Could you check a few things on this model? Use its own coordinates, in mm. Coordinates: 2 decimals unless noted, no trailing zeros. Loops run counter-clockwise (first coordinate to the right, second up) from the corner with the lowest first, then second, coordinate; pieces in that order, holes last. Notation, with made-up numbers: M 56.25,89.5 L 69.25,89.5 A31 ccw 69.25,120.5 Z; hole C 88.25,33 d3. An arc over 180 degrees is marked long. Use one line per item in the form item = value. Start each with the question number.
Autodesk Fusion 360 part; units mm, degrees
box "BoxPrimitive1" add length 123 width 170 height 1 placed x (0, -1, 0) y (1, 0, 0) z (0, 0, 1) at (0, 0, 0) makes body 1
cylinder "CylinderPrimitive1" add diameter 5 height 10 placed x (0, 0, -1) y (0, 1, 0) z (1, 0, 0) at (0, 10, 10) separate body makes body 2
move_body "Move1" bodies 2 to x (1, 0, 0) y (0, 1, 0) z (0, 0, 1) at (0, -10, -10)
move_body "Move2" bodies 2 to x (1, 0, 0) y (0, 1, 0) z (0, 0, 1) at (0, -61.5, 0)
move_body "Move3" bodies 2 to x (1, 0, 0) y (0, 1, 0) z (0, 0, 1) at (-5, 0, 0)
combine "Combine1" operation add target body 1 tool bodies 2
cylinder "CylinderPrimitive2" cut diameter 3.5 height -1 placed x (1, 0, 0) y (0, 1, 0) z (0, 0, 1) at (24, -14, 1) bodies 1
Item 1: Thinking about a two-plate mould opening in Y: for faces 1 (the cylindrical face through (22.71, -12.82, 0.51)), 2 (the flat face through (86, -61, 1)), 3 (the cylindrical face through (0.07, -60.749, -2.385)), which applies, pulls with the +Y half, pulls with the -Y half, needs draft (parallel to the pull), parting line crosses it, or undercut?
Item 2: I want a section at C-C (x = 135). Write out the boundary of the cut face in (y, z).
Item 3: Please list where these lines run through material, in increasing order: line 1 along Y through (x, z) = (24, 0.35); line 2 along Z through (x, y) = (60.5, -25); line 3 along X through (y, z) = (-92, 0.3).
Item 4: I want a section at A-A (y = -14). Write out the boundary of the cut face in (x, z).
Item 5: I'm going to push flat-ended pins straight in: P1, Ø0.8, axis at y = -62.5, z = 2, coming from the +X side; P2, Ø5, axis at x = 131.5, y = -84, coming from the -Z side; P3, Ø10, axis at x = 86.5, y = -44, coming from the +Z side. Where does each tip first touch, or does it pass through?
Item 6: I want a section at B-B (x = 24). Write out the boundary of the cut face in (y, z).
Item 7: I want a section at D-D (z = -1.65). Write out the boundary of the cut face in (x, y).
Worked answers:
q1.face_1 = undercut
q1.face_2 = needs draft
q1.face_3 = parting line crosses it
q2.outline = M -123,0 L 0,0 L 0,1 L -123,1 Z
q3.line_1 = -123 to -15.75, -12.25 to 0
q3.line_2 = 0 to 1
q3.line_3 = 0 to 170
q4.outline = M 0,0 L 22.25,0 L 22.25,1 L 0,1 Z; M 25.75,0 L 170,0 L 170,1 L 25.75,1 Z
q5.P1 = 5
q5.P2 = 0
q5.P3 = 1
q6.outline = M -123,0 L -15.75,0 L -15.75,1 L -123,1 Z; M -12.25,0 L 0,0 L 0,1 L -12.25,1 Z
q7.outline = M -5,-63.38 L 5,-63.38 L 5,-59.62 L -5,-59.62 Z
